For this review, take the finished solid that the model builds, in its own axes (mm). Face numbers are marked on the shaded views. A direction names the side the tool comes from. Coordinates: 2 decimals unless noted, no trailing zeros. Write each loop counter-clockwise with the first axis right and the second up, starting at its lowest first coordinate (ties: lowest second). Pieces come first, ordered by that corner, then holes. Notation, with made-up numbers: (-28, 46.5) -> (11, 46.5) arc R7 ccw to (11, 52.5) -> close; hole circle Ø9 at (6.25, -1.75). An arc over 180 degrees is marked (long way). One line per item, written item: value. Start each with the question number.
1) Mouldability with a two-part tool opening along Y and no side actions: class the marked faces 3, 4 and 5 as released by +Y, released by -Y, zero draft, split by the parting line, or undercut.
2) Add section A-A (y = 0). State the section outline as (x, z) points, and give its area (3 significant figures).
3) For pin 1 Ø1.5 at (y, z) = (224, -193.5) entering from +X; pin 2 Ø3 at (y, z) = (101.5, 62.5) entering from -X; pin 3 Ø5 at (y, z) = (-121.5, 66) entering from +X, all flat-tipped, find the tip position at first contact; note any pin that passes through.
4) For probe 1 along Z at (x, y) = (139, -310.5); probe 2 along X at (y, z) = (0, 179), list the stretches that pass through material, from the lowest coordinate up. Write a range as from..to.
5) Add section C-C (z = 232.5). State the section outline as (x, y) points, and give its area (4 significant figures).
6) Machinability: for the marked faces 1 and 2, which of the approach directions +Z, -Z, +X, -X, +Y, -Y give a long, thin tool a straight path to every point of the face, cutting with its end or side? Answer none if there is none.
7) Add section D-D (z = 168). State the section outline as (x, y) points, and give its area (3 significant figures).
from build123d import *

# Parameters (mm, degrees)
F2_R = 30
F3_R = 50
F4_R = 50


with BuildPart() as f1:
    # F0 (on Front) → F1 (revolve)
    with BuildSketch(Plane.XZ):
        Polygon((350, 300), (100, 300), (100, 150), (225, 0), (225, -300), (500, -300), (500, -150), (430, 60), (300, 60), (300, 200), (383.333333, 200), align=None)
    revolve(axis=Axis((0, 0, 0), (0, 0, -1)))

    # F2
    f2_edges = [f1.edges().sort_by_distance(p)[0] for p in [
        (-100, 0, 300),
    ]]
    fillet(f2_edges, radius=F2_R)

    # F3
    f3_edges = [f1.edges().sort_by_distance(p)[0] for p in [
        (-500, 0, -300),
    ]]
    fillet(f3_edges, radius=F3_R)

    # F4
    f4_edges = [f1.edges().sort_by_distance(p)[0] for p in [
        (-225, 0, -300),
    ]]
    fillet(f4_edges, radius=F4_R)


solid = f1.part
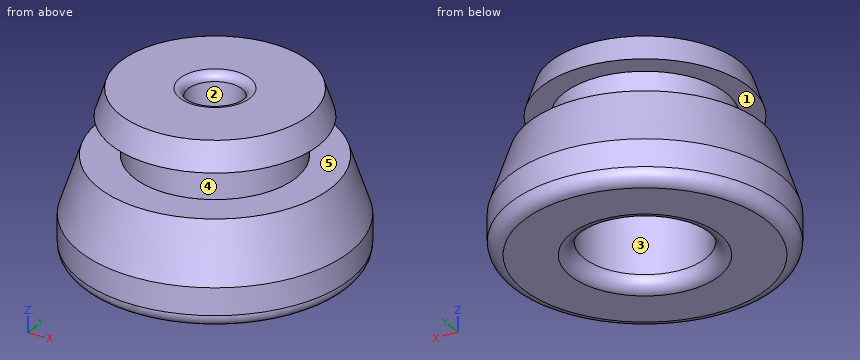
Numbers:
1. face 3: undercut
1. face 4: split by the parting line
1. face 5: zero draft
2. outline: (-500, -250) arc R50 ccw to (-450, -300) -> (-275, -300) arc R50 ccw to (-225, -250) -> (-225, 0) -> (-100, 150) -> (-100, 270) arc R30 ccw to (-130, 300) -> (-350, 300) -> (-383.33, 200) -> (-300, 200) -> (-300, 60) -> (-430, 60) -> (-500, -150) -> close; (100, 150) -> (225, 0) -> (225, -250) arc R50 ccw to (275, -300) -> (450, -300) arc R50 ccw to (500, -250) -> (500, -150) -> (430, 60) -> (300, 60) -> (300, 200) -> (383.33, 200) -> (350, 300) -> (130, 300) arc R30 ccw to (100, 270) -> close
2. area: 286,000 mm²
3. pin 1: x = 447.39
3. pin 2: x = -282.84
3. pin 3: x = 275.39
4. probe 1: -300..60, 200..300
4. probe 2: -300..-100, 100..300
5. outline: circle Ø745 at (0, 0); hole circle Ø200 at (0, 0)
5. area: 404,500 mm²
6. face 1: none
6. face 2: +Z, -Z
7. outline: circle Ø600 at (0, 0); hole circle Ø200 at (0, 0)
7. area: 251,000 mm²
